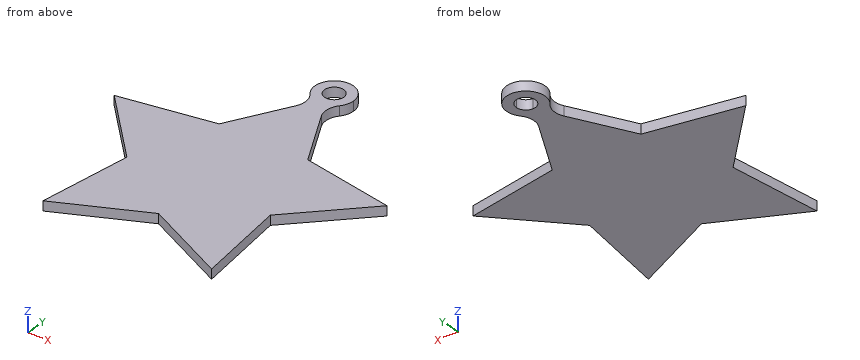
```python
from build123d import *

# Parameters (mm, degrees)
F1_DEPTH = 1


with BuildPart() as f1:
    # F0 (on Top) → F1 (new body)
    with BuildSketch(Plane.XY):
        with BuildLine():
            Line((4.6352549156, 6.3798810626), (1.3339177444, 12.5193317695))
            Line((1.3339177444, 12.5193317695), (0.503138004, 14.0643212692))
            ThreePointArc((0.503138004, 14.0643212692), (0, 14), (-0.503138004, 14.0643212692))
            Line((-0.503138004, 14.0643212692), (-1.3339177444, 12.5193317695))
            Line((-1.3339177444, 12.5193317695), (-4.6352549156, 6.3798810626))
            Line((-4.6352549156, 6.3798810626), (-14.2658477444, 4.6352549156))
            Line((-14.2658477444, 4.6352549156), (-7.5, -2.4368977217))
            Line((-7.5, -2.4368977217), (-8.8167787844, -12.1352549156))
            Line((-8.8167787844, -12.1352549156), (0, -7.8859666818))
            Line((0, -7.8859666818), (8.8167787844, -12.1352549156))
            Line((8.8167787844, -12.1352549156), (7.5, -2.4368977217))
            Line((7.5, -2.4368977217), (14.2658477444, 4.6352549156))
            Line((14.2658477444, 4.6352549156), (4.6352549156, 6.3798810626))
        make_face()
        with BuildLine():
            Line((0.503138004, 14.0643212692), (1.3339177444, 12.5193317695))
            ThreePointArc((1.3339177444, 12.5193317695), (1.1046607275, 13.6587566576), (1.547700554, 14.7332628547))
            ThreePointArc((1.547700554, 14.7332628547), (1.0785895461, 14.315765874), (0.503138004, 14.0643212692))
        make_face()
        with BuildLine():
            ThreePointArc((-0.503138004, 14.0643212692), (0, 14), (0.503138004, 14.0643212692))
            Line((0.503138004, 14.0643212692), (0, 15))
            Line((0, 15), (-0.503138004, 14.0643212692))
        make_face()
        with BuildLine():
            Line((-1.3339177444, 12.5193317695), (-0.503138004, 14.0643212692))
            ThreePointArc((-0.503138004, 14.0643212692), (-1.0785895461, 14.315765874), (-1.547700554, 14.7332628547))
            ThreePointArc((-1.547700554, 14.7332628547), (-1.1046607275, 13.6587566576), (-1.3339177444, 12.5193317695))
        make_face()
        with BuildLine():
            Line((0, 15), (0.503138004, 14.0643212692))
            ThreePointArc((0.503138004, 14.0643212692), (1.0785895461, 14.315765874), (1.547700554, 14.7332628547))
            ThreePointArc((1.547700554, 14.7332628547), (1.8835340597, 15.3274678848), (2, 16))
            ThreePointArc((2, 16), (-0.6725321152, 17.8835340597), (-1.547700554, 14.7332628547))
            ThreePointArc((-1.547700554, 14.7332628547), (-1.0785895461, 14.315765874), (-0.503138004, 14.0643212692))
            Line((-0.503138004, 14.0643212692), (0, 15))
        make_face()
        with BuildLine():
            ThreePointArc((1, 16), (0.7071067812, 15.2928932188), (0, 15))
            ThreePointArc((0, 15), (-0.7071067812, 16.7071067812), (1, 16))
        make_face(mode=Mode.SUBTRACT)
    extrude(amount=F1_DEPTH)


solid = f1.part
```
The listing builds one solid part. Answer for the finished solid, in the listing's coordinates (mm). Give positions to 0.01 mm unless a question says otherwise; leave off trailing zeros. Order: outer loops, then holes, each group sorted by start corner. A loop starts at its lowest first (then second) coordinate and runs counter-clockwise, first axis right, second up.
1) Find section C-C on x = -12. Write down the section's boundary in (y, z).
Reported:
outline: (2.27, 0) - (5.05, 0) - (5.05, 1) - (2.27, 1) - close
2) Find section B-B on y = 10. Write down the section's boundary in (x, z).
Reported:
outline: (-2.69, 0) - (2.69, 0) - (2.69, 1) - (-2.69, 1) - close
3) Consider line 1 along X through (y, z) = (16, 0.35); line 2 along X through (y, z) = (-9, 0.65); line 3 along Y through (x, z) = (0.5, 0.65). Determine where each line is inside the solid, lowest interval first.
Reported:
line 1: x = -2 to -1, 1 to 2
line 2: x = -8.39 to -2.31, 2.31 to 8.39
line 3: y = -8.13 to 15.13, 16.87 to 17.94
4) Find section A-A on z = 0.85. Write down the section's boundary in (x, y).
Reported:
outline: (-14.27, 4.64) - (-7.5, -2.44) - (-8.82, -12.14) - (0, -7.89) - (8.82, -12.14) - (7.5, -2.44) - (14.27, 4.64) - (4.64, 6.38) - (1.33, 12.52) arc R2 cw to (1.55, 14.73) arc R2 ccw (long way) to (-1.55, 14.73) arc R2 cw to (-1.33, 12.52) - (-4.64, 6.38) - close; hole circle Ø2 at (0, 16)
